For this review, take the finished solid that the model builds, in its own axes (mm). Face numbers are marked on the shaded views. A direction names the side the tool comes from. Coordinates: 2 decimals unless noted, no trailing zeros. Loops run counter-clockwise (first coordinate to the right, second up) from the corner with the lowest first, then second, coordinate; pieces in that order, holes last. Notation, with made-up numbers: (52.5, -36) -> (81.5, -36) arc R20 cw to (81.5, -25) -> close; hole circle Ø9 at (6.25, -9.5). An arc over 180 degrees is marked (long way). Answer in a Markdown table with one row per item.
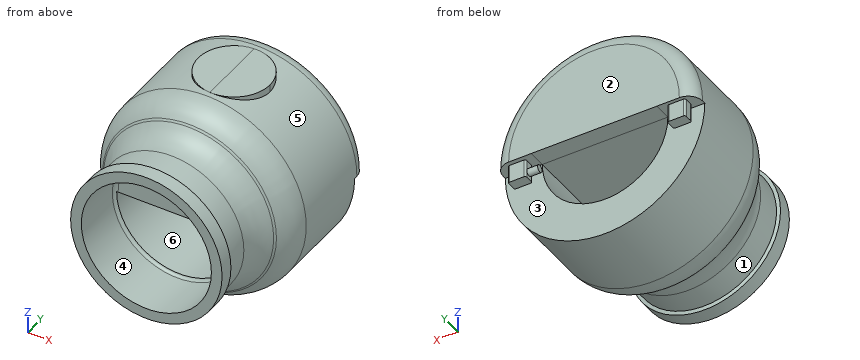
from build123d import *
from build123d.topology import SkipClean

# Parameters (mm, degrees)
SKETCH10_R              = 10
BOSS_EXTRUDE1_DEPTH     = 5
CUT_EXTRUDE3_DEPTH      = 45
CUT_EXTRUDE3_DEPTH_BACK = 20
CUT_EXTRUDE5_DEPTH      = 5
BOSS_EXTRUDE2_DEPTH     = 5
SKETCH14_R              = 1
BOSS_EXTRUDE3_DEPTH     = 3


with BuildPart() as part:
    # Sketch1 → Revolve1 (revolve)
    with BuildSketch(Plane.XY):
        with BuildLine():
            Line((20.9, 0), (23.871591838, 0))
            Line((23.871591838, 0), (23.871591838, 4))
            Line((23.871591838, 4), (22.9, 4.236662843))
            Line((22.9, 4.236662843), (22.9, 11.404308102))
            ThreePointArc((22.9, 11.404308102), (23.83692213, 15.63049072), (26.472123903, 19.064752533))
            Line((26.472123903, 19.064752533), (26.988320528, 19.497892931))
            ThreePointArc((26.988320528, 19.497892931), (29.623522302, 22.932154745), (30.560444431, 27.158337362))
            Line((30.560444431, 27.158337362), (30.560444431, 50))
            ThreePointArc((30.560444431, 50), (29.388871556, 52.828427125), (26.560444431, 54))
            Line((26.560444431, 54), (2.764914955, 54))
            Line((2.764914955, 54), (2.764914955, 15))
            Line((2.764914955, 15), (19.9, 15))
            ThreePointArc((19.9, 15), (20.607106781, 14.707106781), (20.9, 14))
            Line((20.9, 14), (20.9, 0))
        make_face()
    revolve(axis=Axis((2.764914955, 7.821821657, 0), (0, 1, 0)))

    # Sketch10 → Boss-Extrude1 (add)
    with SkipClean():  # the faces are left unmerged after this step: merging them gives an invalid solid
        with BuildSketch(Plane.XY.offset(27.795529476)):
            with Locations((3.346345887, 38.658337362)):
                Circle(SKETCH10_R)
        extrude(amount=-BOSS_EXTRUDE1_DEPTH)

    # Sketch11 → Cut-Extrude3 (cut, two sides: drawn at the far end of the back side and taken through both)
    with SkipClean():  # the faces are left unmerged after this step: merging them gives an invalid solid
        with BuildSketch(Plane(origin=(0, 17, 0), x_dir=(1, 0, 0), z_dir=(0, 1, 0)).offset(-CUT_EXTRUDE3_DEPTH_BACK)):
            with BuildLine():
                Line((-14.735085045, 0), (20.264914955, 0))
                ThreePointArc((20.264914955, 0), (2.764914955, 17.5), (-14.735085045, 0))
            make_face()
        extrude(amount=CUT_EXTRUDE3_DEPTH + CUT_EXTRUDE3_DEPTH_BACK, mode=Mode.SUBTRACT)

    # Sketch9 → Cut-Extrude5 (cut)
    with SkipClean():  # the faces are left unmerged after this step: merging them gives an invalid solid
        with BuildSketch(Plane(origin=(0, 54, 0), x_dir=(1, 0, 0), z_dir=(0, 1, 0))):
            with BuildLine():
                Line((-25.235085045, 0), (30.764914955, 0))
                ThreePointArc((30.764914955, 0), (2.764914955, 28), (-25.235085045, 0))
            make_face()
        extrude(amount=-CUT_EXTRUDE5_DEPTH, mode=Mode.SUBTRACT)

    # Sketch13 → Boss-Extrude2 (add)
    with SkipClean():  # the faces are left unmerged after this step: merging them gives an invalid solid
        with BuildSketch(Plane(origin=(0, 0, 0), x_dir=(-1, 0, 0), z_dir=(0, 0, -1))):
            with BuildLine():
                Line((17.53061452, 53), (21.53061452, 53))
                ThreePointArc((21.53061452, 53), (21.884167911, 52.853553391), (22.03061452, 52.5))
                Line((22.03061452, 52.5), (22.03061452, 50.5))
                ThreePointArc((22.03061452, 50.5), (21.884167911, 50.146446609), (21.53061452, 50))
                Line((21.53061452, 50), (17.53061452, 50))
                ThreePointArc((17.53061452, 50), (17.17706113, 50.146446609), (17.03061452, 50.5))
                Line((17.03061452, 50.5), (17.03061452, 52.5))
                ThreePointArc((17.03061452, 52.5), (17.17706113, 52.853553391), (17.53061452, 53))
            make_face()
            with BuildLine():
                Line((-27.060444431, 52.75), (-23.060444431, 52.75))
                ThreePointArc((-23.060444431, 52.75), (-22.706891041, 52.603553391), (-22.560444431, 52.25))
                Line((-22.560444431, 52.25), (-22.560444431, 50.25))
                ThreePointArc((-22.560444431, 50.25), (-22.706891041, 49.896446609), (-23.060444431, 49.75))
                Line((-23.060444431, 49.75), (-27.060444431, 49.75))
                ThreePointArc((-27.060444431, 49.75), (-27.413997822, 49.896446609), (-27.560444431, 50.25))
                Line((-27.560444431, 50.25), (-27.560444431, 52.25))
                ThreePointArc((-27.560444431, 52.25), (-27.413997822, 52.603553391), (-27.060444431, 52.75))
            make_face()
        extrude(amount=BOSS_EXTRUDE2_DEPTH)

    # Sketch14 → Boss-Extrude3 (add)
    with SkipClean():  # the faces are left unmerged after this step: merging them gives an invalid solid
        with BuildSketch(Plane.ZY.offset(-22.560444431)):
            with Locations(Location((-3, 51.25, 0), (0, 0, 270))):
                Circle(SKETCH14_R)
        extrude(amount=BOSS_EXTRUDE3_DEPTH)


solid = part.part
Item 1: For L1, parallel to X at y = 10.25, z = 0; L2, parallel to X at y = 3, z = 0; L3, parallel to Y at x = 6.5, z = 1, list the stretches that pass through material, from the lowest coordinate up.
Worked answers:
| item | result |
|---|---|
| L1 | -17.37 to -15.37, 20.9 to 22.9 |
| L2 | -18.34 to -15.37, 20.9 to 23.87 |
| L3 | 15 to 54 |
Item 2: Take a section at B-B, the plane y = 9. State the section outline as (x, z) points.
Worked answers:
| item | result |
|---|---|
| outline | circle Ø40.27 at (2.76, 0); hole circle Ø36.27 at (2.76, 0) |
Item 3: The part is to be moulded in two halves that separate along X. For the marked faces 3, 4, 5 and 6, say which applies: +X half, -X half, draft (parallel to the pull), parting line (faces both ways), or undercut.
Worked answers:
| item | result |
|---|---|
| face 3 | draft |
| face 4 | undercut |
| face 5 | parting line |
| face 6 | undercut |
Item 4: Take a section at A-A, the plane y = 39.5. State the section outline as (x, z) points, and give its area (3 significant figures).
Worked answers:
| item | result |
|---|---|
| outline | (-6.62, 26.16) arc R27.8 ccw (long way) to (13.31, 25.72) -> (13.31, 27.8) -> (-6.62, 27.8) -> close; hole (-14.74, 0) arc R17.5 ccw to (20.26, 0) -> close |
| area | 1,960 mm² |
Item 5: Insertion check: pin 1 (4 mm diameter, centred on x = -19.5, y = 52.5, fed in from -Z); pin 2 (1.6 mm diameter, centred on y = 51, z = -1, fed in from -X); pin 3 (5 mm diameter, centred on x = -3, z = 11, fed in from -Y); pin 4 (12 mm diameter, centred on x = 8, z = -19, fed in from -Y). Each pin has a flat end and moves straight along its axis. Give the tip position at first contact, or say it passes through.
Worked answers:
| item | result |
|---|---|
| pin 1 | z = -5 |
| pin 2 | x = -22.03 |
| pin 3 | y = 15 |
| pin 4 | y = 0 |
Item 6: For the marked faces 1 and 2, list the 3-axis set-ups (+Z, -Z, +X, -X, +Y, -Y) from which the entire face can be reached by the end or side of a thin tool; tool diameter is ignored.
Worked answers:
| item | result |
|---|---|
| face 1 | none |
| face 2 | +Z, -Z, +X, -X, +Y |
